Can you work these out from the model? Positions are in its coordinate system, mm. A direction names the side the tool comes from. Round coordinates to 2 decimals unless told otherwise and drop trailing zeros. Loops run counter-clockwise (first coordinate to the right, second up) from the corner with the lowest first, then second, coordinate; pieces in that order, holes last. Notation, with made-up numbers: M 22,87.5 L 55,87.5 A18 ccw 55,92.5 Z; hole C 32.5,76 d6. An arc over 180 degrees is marked long. Use a Markdown table: item, result. Add a question column.
```python
from build123d import *

# Parameters (mm, degrees)
SKETCH1_W               = 914.4
SKETCH1_H               = 9.525
BOSS_EXTRUDE1_DEPTH     = 63.5
SKETCH2_W               = 25.4
SKETCH2_H               = 63.5
CUT_EXTRUDE1_DEPTH      = 6.35
F_1_4_CLEARANCE_HOLE1_D = 6.7564
LPATTERN1_COUNT         = 3
LPATTERN1_PITCH         = 15.875
MIRROR1_COPY_1_D        = 6.7564


with BuildPart() as part:
    # Sketch1 → Boss-Extrude1 (new body)
    with BuildSketch(Plane(origin=(0, 0, 0), x_dir=(1, 0, 0), z_dir=(0, 1, 0))):
        with Locations((0, 4.7625)):
            Rectangle(SKETCH1_W, SKETCH1_H)
    extrude(amount=BOSS_EXTRUDE1_DEPTH)

    # Sketch2 → Cut-Extrude1 (cut)
    with BuildSketch(Plane(origin=(0, 0, -9.525), x_dir=(-1, 0, 0), z_dir=(0, 0, -1))):
        with Locations((-425.45, 31.75)):
            Rectangle(SKETCH2_W, SKETCH2_H)
    cut_extrude1 = extrude(amount=-CUT_EXTRUDE1_DEPTH, mode=Mode.SUBTRACT)

    # 1/4 Clearance Hole1 (through all)
    with Locations(Plane.XY):
        with Locations((425.45, 47.625)):
            f_1_4_clearance_hole1 = Hole(F_1_4_CLEARANCE_HOLE1_D / 2)

    # LPattern1: 1/4 Clearance Hole1 ×3, 1 skipped
    with Locations(*[(0, -i * LPATTERN1_PITCH, 0) for i in range(1, LPATTERN1_COUNT) if i not in (1,)]):
        add(f_1_4_clearance_hole1, mode=Mode.SUBTRACT)

    # Mirror1: Cut-Extrude1, 1/4 Clearance Hole1 across plane
    add(cut_extrude1.mirror(Plane(origin=(0, 0, 0), x_dir=(0, 0, 1), z_dir=(1, 0, 0))), mode=Mode.SUBTRACT)
    add(f_1_4_clearance_hole1.mirror(Plane(origin=(0, 0, 0), x_dir=(0, 0, 1), z_dir=(1, 0, 0))), mode=Mode.SUBTRACT)

    # Mirror1 copy 1 (through all)
    with Locations(Plane(origin=(0, -31.75, 0), x_dir=(-1, 0, 0), z_dir=(0, 0, 1))):
        with Locations((425.45, -47.625)):
            Hole(MIRROR1_COPY_1_D / 2)


solid = part.part
```
(1) Suppose I cut it at A-A on z = -5.5. List the corners of the cut face in (x, y) for me, and give its area (3 significant figures).
(2) I'm going to push flat-ended pins straight in: pin 1 (5.5 mm diameter, centred on x = 425.45, y = 47.625, fed in from -Z); pin 2 (7.5 mm diameter, centred on x = -424, y = 33, fed in from -Z) (3 decimals). Where does each tip first touch, or does it pass through?
(3) On a 3-axis mill with a long thin cutter (end or side, diameter ignored), from which of +Z, -Z, +X, -X, +Y, -Y can I reach the whole of each face in a straight line? I mean faces 1 (the face through (448, 31, -9.525)), 2 (the face through (-426, 32, -3.175)). Say none if no direction works.
(4) Suppose I cut it at B-B on y = 35.5. List the corners of the cut face in (x, z) for me (3 decimals).
(5) Thinking about a two-plate mould opening in X: for faces 3 (the face through (-448, 31, -9.525)), 4 (the face through (426, 32, -3.175)), which applies, released by +X, released by -X, zero draft, split by the parting line, or undercut?
(6) If I drill on probe 1 along X at (y, z) = (6.5, -8.5); probe 2 along Y at (x, z) = (425.45, -2.45); probe 3 along X at (y, z) = (48, -1.75), over which ranges is the centre line in solid material (lowest first)? Write a range as [from, to].
Results below:
| question | item | result |
|---|---|---|
| 1 | outline | M -457.2,0 L -438.15,0 L -438.15,63.5 L -457.2,63.5 Z; M -412.75,0 L 412.75,0 L 412.75,63.5 L -412.75,63.5 Z; M 438.15,0 L 457.2,0 L 457.2,63.5 L 438.15,63.5 Z |
| 1 | area | 54,800 mm² |
| 2 | pin 1 | passes through |
| 2 | pin 2 | stops at z = -3.175 |
| 3 | face 1 | -Z, +X, -X, +Y, -Y |
| 3 | face 2 | -Z, +Y, -Y |
| 4 | outline | M -457.2,-9.525 L -438.15,-9.525 L -438.15,-3.175 L -412.75,-3.175 L -412.75,-9.525 L 412.75,-9.525 L 412.75,-3.175 L 438.15,-3.175 L 438.15,-9.525 L 457.2,-9.525 L 457.2,0 L -457.2,0 Z |
| 5 | face 3 | zero draft |
| 5 | face 4 | undercut |
| 6 | probe 1 | x = [-457.2, -438.15], [-412.75, 412.75], [438.15, 457.2] |
| 6 | probe 2 | y = [0, 12.5], [19.25, 44.25], [51, 63.5] |
| 6 | probe 3 | x = [-457.2, -428.81], [-422.09, 422.09], [428.81, 457.2] |
